Build history of the part. All positions in model axes, mm. Face numbers are marked on the shaded views. A direction names the side the tool comes from. Round coordinates to 2 decimals unless told otherwise and drop trailing zeros. Loops run counter-clockwise (first coordinate to the right, second up) from the corner with the lowest first, then second, coordinate; pieces in that order, holes last. Notation, with made-up numbers: (0.25, 20.25) -> (53.25, 20.25) arc R22 cw to (53.25, 50.25) -> close; hole circle Ø2 at (-20, 42.25). An arc over 180 degrees is marked (long way). Put each result on its own line as item: value. Start each with the question number.
Item 1: Drill centre lines: probe 1 along X at (y, z) = (-0.75, 0); probe 2 along X at (y, z) = (3, 3.75); probe 3 along Z at (x, y) = (-10, -0.5). Where is each one in solid material? Low to high. Write a range as [from, to].
Item 2: Flat gauge pins, fed straight in: pin 1 Ø1 at (y, z) = (4, -1) entering from -X; pin 2 Ø5 at (x, z) = (-8, -1) entering from +Y; pin 3 Ø1.5 at (y, z) = (3.5, 3.5) entering from -X. Where does each tip first touch, or does it go through?
Item 3: Cut at C-C, the plane x = -3.25. List the corners of the cut face in (y, z), plus the area to 3 significant figures.
Item 4: Cut at A-A, the plane z = 0. List the corners of the cut face in (x, y), plus the area to 3 significant figures.
Item 5: Cut at D-D, the plane x = -10. List the corners of the cut face in (y, z).
Item 6: Cut at B-B, the plane y = 0. List the corners of the cut face in (x, z), plus the area to 3 significant figures.
Item 7: Pull direction X, two halves, no side cores. Call the marked faces 3, 4 and 5: +X half, -X half, draft (parallel to the pull), parting line (faces both ways), or undercut.
Item 8: Tool access for the marked faces 1 and 2: list every direction of +Z, -Z, +X, -X, +Y, -Y with a clear straight run to the whole face (end or side of a thin tool).
Autodesk Inventor part; units mm, degrees
ref_plane "YZ Plane" through (0, 0, 0) normal (1, 0, 0) x (0, 1, 0)
ref_plane "XZ Plane" through (0, 0, 0) normal (0, 1, 0) x (-1, 0, 0)
ref_plane "XY Plane" through (0, 0, 0) normal (0, 0, 1) x (1, 0, 0)
sketch "Sketch1" plane through (0, 0, 0) normal (1, 0, 0) x (0, 1, 0)
  circle A0 centre (0, 0) radius 6
  circle A1 centre (0, 0) radius 4.5
  dimension "d0" = 12
  dimension "d1" = 9
extrude "Extrusion1" add sketch "Sketch1" along normal blind 10 contours A0 | A1
extrude "Extrusion2" add sketch "Sketch1" against normal blind 13 contours A1
chamfer "Chamfer1" distance 1 angle 45 1 edges at (-13, -4.5, 0)
thread "Thread1"
sketch "Sketch2" plane through (-13, 0, 0) normal (-1, 0, 0) x (0, 0, 1)
  line L0 (0, 0) -> (-8.2207, 0)
ref_plane "Work Plane1" through (-13, 0, 0) normal (0, 1, 0) x (0, 0, -1)
sketch "Sketch3" plane through (-13, 0, 0) normal (0, 1, 0) x (0, 0, -1)
  circle A0 centre (0, -3) radius 1.5
  line L0 (6, -13) -> (-6, -13)
  point P0 (0, -13)
  dimension "d12" = 3
  dimension "d13" = 10
extrude "Extrusion3" cut sketch "Sketch3" along normal blind 10 and the other way blind 5
properties part number "Tengely"
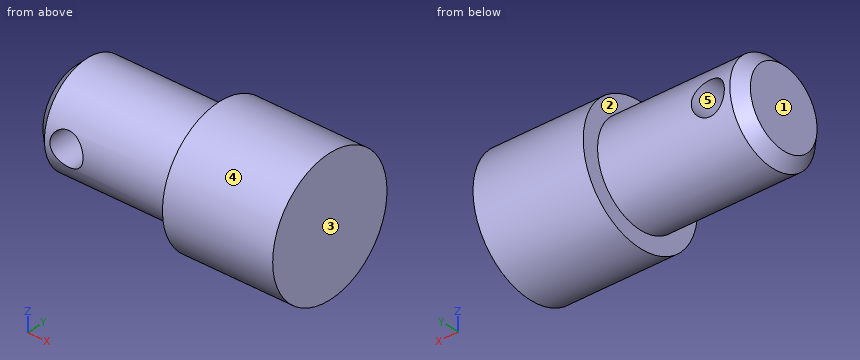
Reply:
1. probe 1: x = [-13, -11.5], [-8.5, 10]
1. probe 2: x = [0, 10]
1. probe 3: z = [-4.47, -1.5], [1.5, 4.47]
2. pin 1: stops at x = -12.88
2. pin 2: stops at y = 4.5
2. pin 3: stops at x = -12.3
3. outline: circle Ø9 at (0, 0)
3. area: 63.6 mm^2
4. outline: (-13, -3.5) -> (-12, -4.5) -> (-11.5, -4.5) -> (-11.5, 4.5) -> (-12, 4.5) -> (-13, 3.5) -> close; (-8.5, -4.5) -> (0, -4.5) -> (0, -6) -> (10, -6) -> (10, 6) -> (0, 6) -> (0, 4.5) -> (-8.5, 4.5) -> close
4. area: 209 mm^2
5. outline: (-4.24, -1.5) arc R4.5 ccw to (4.24, -1.5) -> close; (-4.24, 1.5) -> (4.24, 1.5) arc R4.5 ccw to start
6. outline: (-13, -3.5) -> (-12, -4.5) -> (0, -4.5) -> (0, -6) -> (10, -6) -> (10, 6) -> (0, 6) -> (0, 4.5) -> (-12, 4.5) -> (-13, 3.5) -> close; hole circle Ø3 at (-10, 0)
6. area: 229 mm^2
7. face 3: +X half
7. face 4: draft
7. face 5: undercut
8. face 1: +Z, -Z, -X, +Y, -Y
8. face 2: -X
